Read the model definition and answer for the solid it produces. Units are mm, in the model's axes. A direction names the side the tool comes from. Give positions to 0.01 mm unless a question says otherwise; leave off trailing zeros. Write each loop counter-clockwise with the first axis right and the second up, starting at its lowest first coordinate (ties: lowest second). Pieces come first, ordered by that corner, then holes. Notation, with made-up numbers: (15, 23.5) -> (36, 23.5) arc R19 cw to (36, 38.5) -> close; hole circle Ø10 at (5, 15). An arc over 180 degrees is marked (long way). Write item = value, one per line.
from build123d import *

# Parameters (mm, degrees)
BOSS_EXTRUDE1_DEPTH   = 5
BOSS_EXTRUDE1_2_DEPTH = 5
BOSS_EXTRUDE1_3_DEPTH = 5
BOSS_EXTRUDE1_4_DEPTH = 5
BOSS_EXTRUDE2_DEPTH   = 10
BOSS_EXTRUDE3_DEPTH   = 6
BOSS_EXTRUDE4_DEPTH   = 10


with BuildPart() as part:
    # Sketch1 → Boss-Extrude1 (new, symmetric)
    with BuildSketch(Plane.XY):
        with BuildLine():
            Line((-10, 89), (-10, 54.083269132))
            Line((-10, 54.083269132), (-10, 42.848570571))
            ThreePointArc((-10, 42.848570571), (0, 44), (10, 42.848570571))
            Line((10, 42.848570571), (10, 54.083269132))
            Line((10, 54.083269132), (10, 89))
            Line((10, 89), (10, 95.679491924))
            ThreePointArc((10, 95.679491924), (0, 93), (-10, 95.679491924))
            Line((-10, 95.679491924), (-10, 89))
        make_face()
    extrude(amount=BOSS_EXTRUDE1_DEPTH, both=True)



with BuildPart() as body_2:
    # Sketch1 → Boss-Extrude1 2 (new, symmetric)
    with BuildSketch(Plane.XY):
        with BuildLine():
            Line((-89, 10), (-95.679491924, 10))
            ThreePointArc((-95.679491924, 10), (-93.681483474, 5.176380902), (-93, 0))
            ThreePointArc((-93, 0), (-93.681483474, -5.176380902), (-95.679491924, -10))
            Line((-95.679491924, -10), (-89, -10))
            Line((-89, -10), (-54.083269132, -10))
            Line((-54.083269132, -10), (-42.848570571, -10))
            ThreePointArc((-42.848570571, -10), (-44, 0), (-42.848570571, 10))
            Line((-42.848570571, 10), (-54.083269132, 10))
            Line((-54.083269132, 10), (-89, 10))
        make_face()
    extrude(amount=BOSS_EXTRUDE1_2_DEPTH, both=True)


with BuildPart() as body_3:
    # Sketch1 → Boss-Extrude1 3 (new, symmetric)
    with BuildSketch(Plane.XY):
        with BuildLine():
            Line((54.083269132, 10), (42.848570571, 10))
            ThreePointArc((42.848570571, 10), (43.71119482, 5.033035608), (44, 0))
            ThreePointArc((44, 0), (43.71119482, -5.033035608), (42.848570571, -10))
            Line((42.848570571, -10), (54.083269132, -10))
            Line((54.083269132, -10), (89, -10))
            Line((89, -10), (95.679491924, -10))
            ThreePointArc((95.679491924, -10), (93, 0), (95.679491924, 10))
            Line((95.679491924, 10), (89, 10))
            Line((89, 10), (54.083269132, 10))
        make_face()
    extrude(amount=BOSS_EXTRUDE1_3_DEPTH, both=True)


with BuildPart() as body_4:
    # Sketch1 → Boss-Extrude1 4 (new, symmetric)
    with BuildSketch(Plane.XY):
        with BuildLine():
            Line((-10, -42.848570571), (-10, -54.083269132))
            Line((-10, -54.083269132), (-10, -89))
            Line((-10, -89), (-10, -95.679491924))
            ThreePointArc((-10, -95.679491924), (0, -93), (10, -95.679491924))
            Line((10, -95.679491924), (10, -89))
            Line((10, -89), (10, -54.083269132))
            Line((10, -54.083269132), (10, -42.848570571))
            ThreePointArc((10, -42.848570571), (0, -44), (-10, -42.848570571))
        make_face()
    extrude(amount=BOSS_EXTRUDE1_4_DEPTH, both=True)


with BuildPart() as part_1:
    add(part.part)

    add(body_2.part)  # Boss-Extrude2 merges body 2

    add(body_3.part)  # Boss-Extrude2 merges body 3

    add(body_4.part)  # Boss-Extrude2 merges body 4
    # Sketch1_3 → Boss-Extrude2 (add, symmetric)
    with BuildSketch(Plane.XY):
        with BuildLine():
            ThreePointArc((-10, 54.083269132), (-38.890872965, 38.890872965), (-54.083269132, 10))
            Line((-54.083269132, 10), (-42.848570571, 10))
            ThreePointArc((-42.848570571, 10), (-31.112698372, 31.112698372), (-10, 42.848570571))
            Line((-10, 42.848570571), (-10, 54.083269132))
        make_face()
        with BuildLine():
            Line((10, 54.083269132), (10, 42.848570571))
            ThreePointArc((10, 42.848570571), (31.112698372, 31.112698372), (42.848570571, 10))
            Line((42.848570571, 10), (54.083269132, 10))
            ThreePointArc((54.083269132, 10), (38.890872965, 38.890872965), (10, 54.083269132))
        make_face()
        with BuildLine():
            ThreePointArc((42.848570571, -10), (31.112698372, -31.112698372), (10, -42.848570571))
            Line((10, -42.848570571), (10, -54.083269132))
            ThreePointArc((10, -54.083269132), (38.890872965, -38.890872965), (54.083269132, -10))
            Line((54.083269132, -10), (42.848570571, -10))
        make_face()
        with BuildLine():
            Line((-42.848570571, -10), (-54.083269132, -10))
            ThreePointArc((-54.083269132, -10), (-38.890872965, -38.890872965), (-10, -54.083269132))
            Line((-10, -54.083269132), (-10, -42.848570571))
            ThreePointArc((-10, -42.848570571), (-31.112698372, -31.112698372), (-42.848570571, -10))
        make_face()
    extrude(amount=BOSS_EXTRUDE2_DEPTH, both=True)

    # Sketch1_4 → Boss-Extrude3 (add, symmetric)
    with BuildSketch(Plane.XY):
        with BuildLine():
            ThreePointArc((-131.384776311, 18.384776311), (-107.954328319, 25.505709112), (-89, 10))
            Line((-89, 10), (-54.083269132, 10))
            ThreePointArc((-54.083269132, 10), (-38.890872965, 38.890872965), (-10, 54.083269132))
            Line((-10, 54.083269132), (-10, 89))
            ThreePointArc((-10, 89), (-25.505709112, 107.954328319), (-18.384776311, 131.384776311))
            Line((-18.384776311, 131.384776311), (-131.384776311, 18.384776311))
        make_face()
        with BuildLine():
            Line((131.384776311, 18.384776311), (18.384776311, 131.384776311))
            ThreePointArc((18.384776311, 131.384776311), (25.505709112, 107.954328319), (10, 89))
            Line((10, 89), (10, 54.083269132))
            ThreePointArc((10, 54.083269132), (38.890872965, 38.890872965), (54.083269132, 10))
            Line((54.083269132, 10), (89, 10))
            ThreePointArc((89, 10), (107.954328319, 25.505709112), (131.384776311, 18.384776311))
        make_face()
        with BuildLine():
            ThreePointArc((52.359428182, -36.803400392), (74.773631801, -21.15717706), (102.002815768, -23.559752524))
            ThreePointArc((102.002815768, -23.559752524), (94.233874983, -17.995348061), (89, -10))
            Line((89, -10), (54.083269132, -10))
            ThreePointArc((54.083269132, -10), (38.890872965, -38.890872965), (10, -54.083269132))
            Line((10, -54.083269132), (10, -89))
            ThreePointArc((10, -89), (17.995348061, -94.233874983), (23.559752524, -102.002815768))
            ThreePointArc((23.559752524, -102.002815768), (21.15717706, -74.773631801), (36.803400392, -52.359428182))
            ThreePointArc((36.803400392, -52.359428182), (45.254833996, -45.254833996), (52.359428182, -36.803400392))
        make_face()
        with BuildLine():
            Line((-54.083269132, -10), (-89, -10))
            ThreePointArc((-89, -10), (-94.233874983, -17.995348061), (-102.002815768, -23.559752524))
            ThreePointArc((-102.002815768, -23.559752524), (-74.773631801, -21.15717706), (-52.359428182, -36.803400392))
            ThreePointArc((-52.359428182, -36.803400392), (-45.254833996, -45.254833996), (-36.803400392, -52.359428182))
            ThreePointArc((-36.803400392, -52.359428182), (-21.15717706, -74.773631801), (-23.559752524, -102.002815768))
            ThreePointArc((-23.559752524, -102.002815768), (-17.995348061, -94.233874983), (-10, -89))
            Line((-10, -89), (-10, -54.083269132))
            ThreePointArc((-10, -54.083269132), (-38.890872965, -38.890872965), (-54.083269132, -10))
        make_face()
    extrude(amount=BOSS_EXTRUDE3_DEPTH, both=True)

    # Sketch1_5 → Boss-Extrude4 (add, symmetric)
    with BuildSketch(Plane.XY):
        with BuildLine():
            ThreePointArc((18.384776311, 131.384776311), (0, 139), (-18.384776311, 131.384776311))
            ThreePointArc((-18.384776311, 131.384776311), (-25.505709112, 107.954328319), (-10, 89))
            Line((-10, 89), (-10, 95.679491924))
            ThreePointArc((-10, 95.679491924), (-10, 130.320508076), (20, 113))
            ThreePointArc((20, 113), (17.320508076, 103), (10, 95.679491924))
            Line((10, 95.679491924), (10, 89))
            ThreePointArc((10, 89), (25.505709112, 107.954328319), (18.384776311, 131.384776311))
        make_face()
        with BuildLine():
            ThreePointArc((-95.679491924, -10), (-133, 0), (-95.679491924, 10))
            Line((-95.679491924, 10), (-89, 10))
            ThreePointArc((-89, 10), (-107.954328319, 25.505709112), (-131.384776311, 18.384776311))
            ThreePointArc((-131.384776311, 18.384776311), (-134.295069945, -14.917104144), (-102.002815768, -23.559752524))
            ThreePointArc((-102.002815768, -23.559752524), (-94.233874983, -17.995348061), (-89, -10))
            Line((-89, -10), (-95.679491924, -10))
        make_face()
        with BuildLine():
            ThreePointArc((102.002815768, -23.559752524), (134.295069945, -14.917104144), (131.384776311, 18.384776311))
            ThreePointArc((131.384776311, 18.384776311), (107.954328319, 25.505709112), (89, 10))
            Line((89, 10), (95.679491924, 10))
            ThreePointArc((95.679491924, 10), (118.176380902, 19.318516526), (133, 0))
            ThreePointArc((133, 0), (118.176380902, -19.318516526), (95.679491924, -10))
            Line((95.679491924, -10), (89, -10))
            ThreePointArc((89, -10), (94.233874983, -17.995348061), (102.002815768, -23.559752524))
        make_face()
        with BuildLine():
            Line((-10, -95.679491924), (-10, -89))
            ThreePointArc((-10, -89), (-17.995348061, -94.233874983), (-23.559752524, -102.002815768))
            ThreePointArc((-23.559752524, -102.002815768), (0, -139), (23.559752524, -102.002815768))
            ThreePointArc((23.559752524, -102.002815768), (17.995348061, -94.233874983), (10, -89))
            Line((10, -89), (10, -95.679491924))
            ThreePointArc((10, -95.679491924), (17.320508076, -103), (20, -113))
            ThreePointArc((20, -113), (-10, -130.320508076), (-10, -95.679491924))
        make_face()
    extrude(amount=BOSS_EXTRUDE4_DEPTH, both=True)


solid = part_1.part
(1) The part is cut by section B-B on x = 113. Determine the outline of the cut face in (y, z), plus the area to 3 significant figures.
Checks:
outline = (-26, -10) -> (-20, -10) -> (-20, 10) -> (-26, 10) -> close; (20, -10) -> (26, -10) -> (26, -6) -> (36.77, -6) -> (36.77, 6) -> (26, 6) -> (26, 10) -> (20, 10) -> close
area = 369 mm²
(2) Consider L1, parallel to Y at x = 113, z = 1.25; L2, parallel to X at y = 6, z = -2.75; L3, parallel to X at y = 22.5, z = -7.5. Determine where each line is inside the solid, lowest interval first.
Checks:
L1 = -26 to -20, 20 to 36.77
L2 = -138.3 to -132.08, -93.92 to -43.59, 43.59 to 93.92, 132.08 to 138.3
L3 = -126.03 to -99.97, -50.19 to -37.81, 37.81 to 50.19, 99.97 to 126.03
(3) A tool of negligible diameter and unlimited length cuts with its end or side. For faces 4 (the cylindrical face through (38.56, -39.22, 7.97)), 5 (the flat face through (5.7, -132.4, -10)), 6 (the cylindrical face through (38.56, -39.22, -8.03)), from which of +Z, -Z, +X, -X, +Y, -Y can it reach the whole face along a straight path? Write none if from no direction.
Checks:
face_4 = +Z
face_5 = -Z, +X, -X, +Y, -Y
face_6 = -Z
(4) The part is cut by section A-A on x = 0. Determine the outline of the cut face in (y, z), plus the area to 3 significant figures.
Checks:
outline = (-139, -10) -> (-133, -10) -> (-133, 10) -> (-139, 10) -> close; (-93, -5) -> (-44, -5) -> (-44, 5) -> (-93, 5) -> close; (44, -5) -> (93, -5) -> (93, 5) -> (44, 5) -> close; (133, -10) -> (139, -10) -> (139, 10) -> (133, 10) -> close
area = 1,220 mm²
(5) For a pull along X with two mould halves and no side action, classify faces 1 (the flat face through (0, 70, -5)), 2 (the cylindrical face through (-45.36, -45.15, 0.08)), 3 (the flat face through (-34, -34, 10)) as released by +X, released by -X, zero draft, split by the parting line, or undercut.
Checks:
face_1 = undercut
face_2 = released by -X
face_3 = zero draft
(6) The part is cut by section C-C on y = 36. Determine the outline of the cut face in (x, z).
Checks:
outline = (-113.77, -6) -> (-41.58, -6) -> (-41.58, -10) -> (-25.3, -10) -> (-25.3, 10) -> (-41.58, 10) -> (-41.58, 6) -> (-113.77, 6) -> close; (25.3, -10) -> (41.58, -10) -> (41.58, -6) -> (113.77, -6) -> (113.77, 6) -> (41.58, 6) -> (41.58, 10) -> (25.3, 10) -> close
(7) Given P1, Ø2, axis at y = -109.5, z = 4.5, coming from the +X side; P2, Ø4, axis at x = -56.5, z = -7.5, coming from the -Y side; P3, Ø4, axis at x = -91.5, z = -8.5, coming from the -Y side; P4, Ø16, axis at x = -5, y = 59.5, coming from the -Z side, each flat-ended and moving along its own axis, determine where each tip first touches the part or whether it passes through.
Checks:
P1 = 25.88
P2 = -33.24
P3 = -17.2
P4 = -10
(8) The part is cut by section D-D on y = 82. Determine the outline of the cut face in (x, z).
Checks:
outline = (-67.77, -6) -> (-10, -6) -> (-10, -5) -> (10, -5) -> (10, -6) -> (67.77, -6) -> (67.77, 6) -> (10, 6) -> (10, 5) -> (-10, 5) -> (-10, 6) -> (-67.77, 6) -> close
